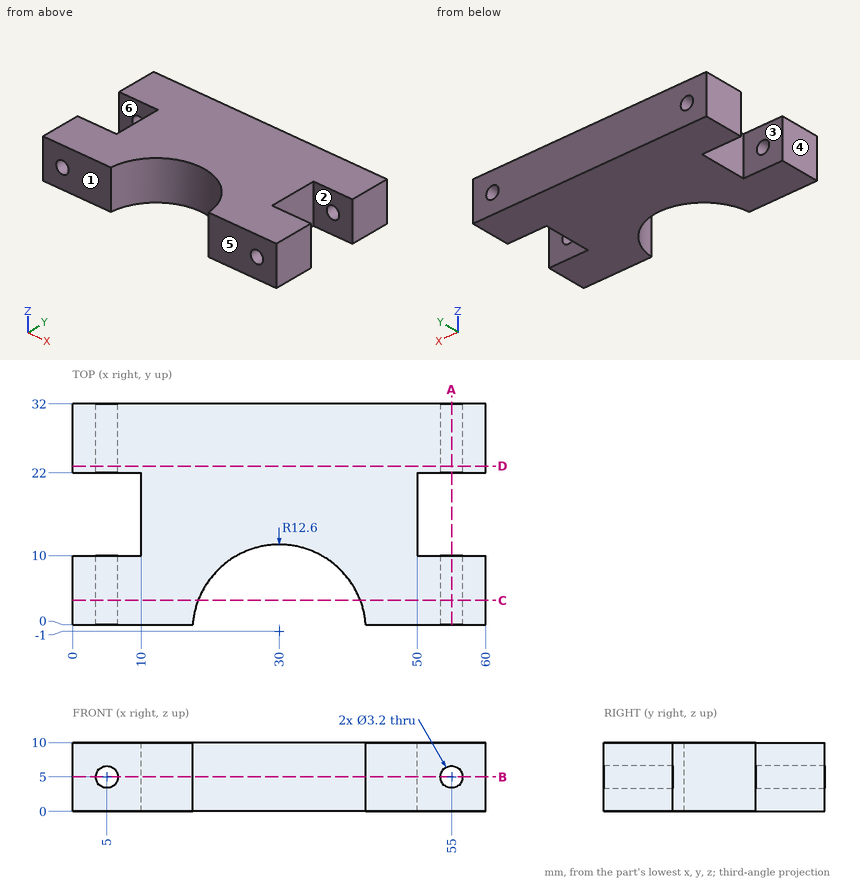
Design review of the part shown in the three views and the two pictorial views. Dimensions are in mm from the part's minimum x, y and z. A direction names the side the tool comes from. Round coordinates to 2 decimals unless told otherwise and drop trailing zeros. Write each loop counter-clockwise with the first axis right and the second up, starting at its lowest first coordinate (ties: lowest second). Pieces come first, ordered by that corner, then holes. Notation, with made-up numbers: (47.5, 72.25) - (84.5, 72.25) arc R19 ccw to (84.5, 80.25) - close; hole circle Ø3 at (25, -20). An arc over 180 degrees is marked (long way). Write item = value, one per line. Start each with the question number.
1. Wall thickness on L1, parallel to Y at x = 8, z = 7.5; L2, parallel to Z at x = 55, y = 30; L3, parallel to X at y = 26.5, z = 4.5: over which ranges is each line inside the solid? List them lowest first.
2. Consider section D-D on y = 23. State the section outline as (x, z) points.
3. Consider section B-B on z = 5. Give the number of separate pieces and of enclosed holes in the cut face, plus the area to 3 significant figures.
4. For the marked faces 1, 2 and 3, list the 3-axis set-ups (+Z, -Z, +X, -X, +Y, -Y) from which the entire face can be reached by the end or side of a thin tool; tool diameter is ignored.
5. Draft analysis for pull direction Y (two halves, no side actions). For the marked faces 4, 5 and 6, state which applies: released by +Y, released by -Y, zero draft, split by the parting line, or undercut.
6. Consider section C-C on y = 3.5. State the section outline as (x, z) points, plus the area to 3 significant figures.
7. For pin 1 Ø1.5 at (y, z) = (19.5, 5) entering from -X; pin 2 Ø5 at (y, z) = (15.5, 7) entering from +X, all flat-tipped, find the tip position at first contact; note any pin that passes through.
8. Consider section A-A on x = 55. State the section outline as (y, z) points, plus the area to 3 significant figures.
Evaluation:
q1.L1 = 0 to 10, 22 to 32
q1.L2 = 0 to 3.4, 6.6 to 10
q1.L3 = 0 to 3.48, 6.52 to 53.48, 56.52 to 60
q2.outline = (0, 0) - (60, 0) - (60, 10) - (0, 10) - close; hole circle Ø3.2 at (5, 5); hole circle Ø3.2 at (55, 5)
q3.separate_pieces = 5
q3.enclosed_holes = 0
q3.area = 1,330 mm2
q4.face_1 = +Z, -Z, +X, -X, -Y
q4.face_2 = +Z, -Z, +X
q4.face_3 = +Z, -Z, -X
q5.face_4 = zero draft
q5.face_5 = released by -Y
q5.face_6 = undercut
q6.outline = (0, 0) - (18.23, 0) - (18.23, 10) - (0, 10) - close; (41.77, 0) - (60, 0) - (60, 10) - (41.77, 10) - close; hole circle Ø3.2 at (5, 5); hole circle Ø3.2 at (55, 5)
q6.area = 349 mm2
q7.pin_1 = 10
q7.pin_2 = 50
q8.outline = (0, 0) - (10, 0) - (10, 3.4) - (0, 3.4) - close; (0, 6.6) - (10, 6.6) - (10, 10) - (0, 10) - close; (22, 0) - (32, 0) - (32, 3.4) - (22, 3.4) - close; (22, 6.6) - (32, 6.6) - (32, 10) - (22, 10) - close
q8.area = 136 mm2
